Input: part model. Units: mm. Frame: model coordinates. Face numbers are marked on the shaded views. A direction names the side the tool comes from. Give positions to 0.01 mm unless a question says otherwise; leave off trailing zeros. Loops run counter-clockwise (first coordinate to the right, second up) from the corner with the lowest first, then second, coordinate; pieces in that order, holes last. Notation, with made-up numbers: (-11, 53.25) -> (7, 53.25) arc R20 cw to (7, 59.25) -> close; hole circle Ø1 at (72.25, 15.5). An arc over 180 degrees is marked (long way). Answer as a JSON object with one key per item and string values.
```python
from build123d import *

# Parameters (mm, degrees)
F0_W     = 25.4762
F0_H     = 19.05
F1_DEPTH = 25.4
F2_DEPTH = 63.5
F3_DEPTH = 7.9375
F5_R     = 6.35


# Not quite as in the source:
# - a feature names something its author has since deleted; it is built from what else it names


with BuildPart() as f1:
    # F0 (on Front) → F1 (new body, symmetric)
    with BuildSketch(Plane.XZ):
        with BuildLine():
            Line((22.225, 9.525), (41.275, 9.525))
            Line((41.275, 9.525), (41.275, 27.0002))
            ThreePointArc((41.275, 27.0002), (45.9246798487, 38.2255201513), (57.15, 42.8752))
            Line((57.15, 42.8752), (60.325, 42.8752))
            Line((60.325, 42.8752), (60.325, 61.9252))
            Line((60.325, 61.9252), (57.15, 61.9252))
            ThreePointArc((57.15, 61.9252), (32.4542956671, 51.6959043329), (22.225, 27.0002))
            Line((22.225, 27.0002), (22.225, 9.525))
        make_face()
        with Locations((73.0631, 52.4002)):
            Rectangle(F0_W, F0_H)
    extrude(amount=F1_DEPTH, both=True)

    # F0 (on Front) → F2 (join, symmetric)
    with BuildSketch(Plane.XZ):
        Polygon((41.275, -9.525), (41.275, 9.525), (22.225, 9.525), (-41.275, 9.525), (-41.275, -9.525), align=None)
    extrude(amount=F2_DEPTH, both=True)

    # F0 (on Front) → F3 (join, symmetric)
    with BuildSketch(Plane.XZ):
        with BuildLine():
            Line((-41.275, 9.525), (22.225, 9.525))
            Line((22.225, 9.525), (22.225, 27.0002))
            ThreePointArc((22.225, 27.0002), (32.4542956671, 51.6959043329), (57.15, 61.9252))
            add(Edge.make_bspline(
                [(-41.275, 9.525), (-40.9908369184, 30.6630749255), (45.7423105836, 66.1747902632), (57.15, 61.9252)],
                knots=[0, 0, 0, 0, 111.5045361635, 111.5045361635, 111.5045361635, 111.5045361635], degree=3))
        make_face()
    extrude(amount=F3_DEPTH, both=True)

    # F0 (on Front) → F4 (revolve)
    with BuildSketch(Plane.XZ):
        Polygon((85.8012, 61.9252), (85.8012, 42.8752), (85.8012, 38.1), (111.125, 38.1), (111.125, 66.675), (85.8012, 66.675), align=None)
    revolve(axis=Axis((85.8012, 0, 52.3875), (0, 0, -1)))

    # F5
    f5_edges = [f1.edges().sort_by_distance(p)[0] for p in [
        (41.275, -63.5, 0),
        (-41.275, -63.5, 0),
        (41.275, 63.5, 0),
        (-41.275, 63.5, 0),
    ]]
    fillet(f5_edges, radius=F5_R)


solid = f1.part
```
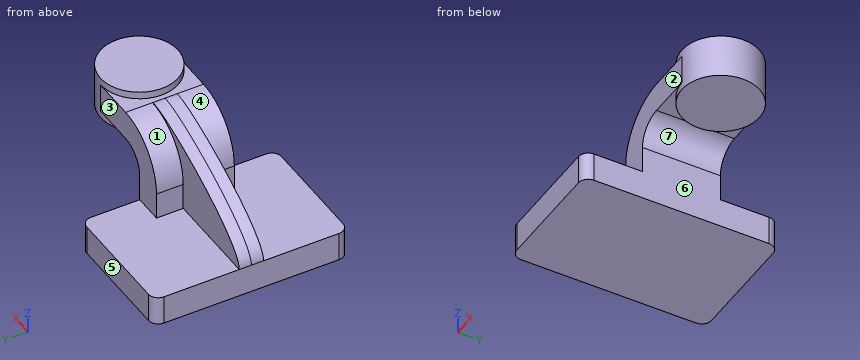
Q1. Section D-D, the plane x = 100. Return the cut outline in (y, z) (3 decimals).
Evaluation:
{"outline": "(-20.969, 38.1) -> (20.969, 38.1) -> (20.969, 66.675) -> (-20.969, 66.675) -> close"}
Q2. Pin query (flat end, axial travel): pin 1 (14 mm diameter, centred on y = -17, z = 18, fed in from -X) (3 decimals); pin 2 (18.5 mm diameter, centred on y = -9, z = 9, fed in from +X) (3 decimals); pin 3 (15.5 mm diameter, centred on x = 42.5, z = 32.5, fed in from +Y). Return the tip coordinate at first contact, or that it passes through.
Evaluation:
{"pin 1": "stops at x = 22.225", "pin 2": "stops at x = 41.275", "pin 3": "stops at y = 25.4"}
Q3. Section A-A, the plane z = 7.5. Return the cut outline in (x, y) (3 decimals).
Evaluation:
{"outline": "(-41.275, -57.15) arc R6.35 ccw to (-34.925, -63.5) -> (34.925, -63.5) arc R6.35 ccw to (41.275, -57.15) -> (41.275, 57.15) arc R6.35 ccw to (34.925, 63.5) -> (-34.925, 63.5) arc R6.35 ccw to (-41.275, 57.15) -> close"}
Q4. Section B-B, the plane y = 52. Return the cut outline in (x, z) (3 decimals), then the cut area to 3 significant figures.
Evaluation:
{"outline": "(-41.275, -9.525) -> (41.275, -9.525) -> (41.275, 9.525) -> (-41.275, 9.525) -> close", "area": "1,570 mm2"}
Q5. Access query for the marked faces 1, 2 and 3. Directions: +Z, -Z, +X, -X, +Y, -Y. A direction counts if a zero-diameter tool reaches every point of the face in a straight line with its end or side. Return the directions, or none.
Evaluation:
{"face 1": "+Z, -X, +Y", "face 2": "+Z, +X, -X, -Y", "face 3": "+Z, +X, -X, +Y"}
Q6. Draft query along X for the marked faces 4, 5, 6 and 7. Return one class per face: +X half, -X half, draft (parallel to the pull), parting line (faces both ways), or undercut.
Evaluation:
{"face 4": "-X half", "face 5": "draft", "face 6": "+X half", "face 7": "undercut"}
Q7. Section C-C, the plane x = 65.5. Return the cut outline in (y, z) (3 decimals).
Evaluation:
{"outline": "(-25.4, 42.875) -> (-15.138, 42.875) -> (-15.138, 38.1) -> (15.138, 38.1) -> (15.138, 42.875) -> (25.4, 42.875) -> (25.4, 61.925) -> (15.138, 61.925) -> (15.138, 66.675) -> (-15.138, 66.675) -> (-15.138, 61.925) -> (-25.4, 61.925) -> close"}
Q8. Ray query, line 1 along Y through (x, z) = (-2, 37); line 2 along X through (y, z) = (45, -4.5) (3 decimals); line 3 along Y through (x, z) = (64.5, 43). Return the intervals inside material, ascending.
Evaluation:
{"line 1": "y = -7.94 to 7.94", "line 2": "x = -41.275 to 41.275", "line 3": "y = -25.4 to 25.4"}
